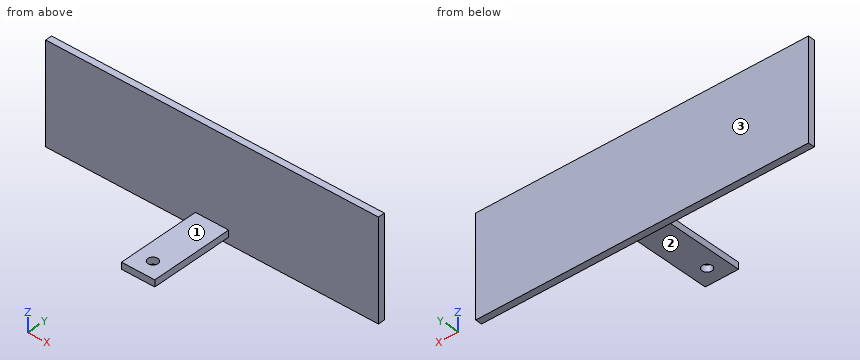
```python
from build123d import *

# Parameters (mm, degrees)
SKETCH1_W               = 2
SKETCH1_H               = 25
BOSS_EXTRUDE1_DEPTH     = 5
BOSS_EXTRUDE2_DEPTH     = 50
CUT_EXTRUDE1_DEPTH      = 64.348243859
CUT_EXTRUDE1_DEPTH_BACK = 64.348243859
SKETCH2_R               = 1.5


with BuildPart() as part:
    # Sketch1 → Boss-Extrude1 (new, symmetric)
    with BuildSketch(Plane(origin=(0, 0, 0), x_dir=(0, 0, -1), z_dir=(1, 0, 0))):
        with Locations((-1, 12.5)):
            Rectangle(SKETCH1_W, SKETCH1_H)
        Polygon((-2, 25), (-28, 25), (-28, 27), (2, 27), (2, 25), (0, 25), align=None)
    extrude(amount=BOSS_EXTRUDE1_DEPTH, both=True)

    # Sketch1_3 → Boss-Extrude2 (add, symmetric)
    with BuildSketch(Plane(origin=(0, 0, 0), x_dir=(0, 0, -1), z_dir=(1, 0, 0))):
        Polygon((-2, 25), (0, 25), (2, 25), (2, 27), (-28, 27), (-28, 25), align=None)
    extrude(amount=BOSS_EXTRUDE2_DEPTH, both=True)

    # Sketch2 → Cut-Extrude1 (cut, two sides: drawn at the far end of the back side and taken through both)
    with BuildSketch(Plane(origin=(0, 0, 0), x_dir=(-1, 0, 0), z_dir=(0, 0, -1)).offset(-CUT_EXTRUDE1_DEPTH_BACK)):
        with Locations((0, 5)):
            Circle(SKETCH2_R)
    extrude(amount=CUT_EXTRUDE1_DEPTH + CUT_EXTRUDE1_DEPTH_BACK, mode=Mode.SUBTRACT)


solid = part.part
```
CAD build for the part. Positions are in the model's coordinates, mm. Face numbers are marked on the shaded views. A direction names the side the tool comes from. Round coordinates to 2 decimals unless told otherwise and drop trailing zeros. Loops run counter-clockwise (first coordinate to the right, second up) from the corner with the lowest first, then second, coordinate; pieces in that order, holes last. Notation, with made-up numbers: M 55.5,-30 L 104.5,-30 A23 cw 104.5,5 Z; hole C -10,-34 d3. An arc over 180 degrees is marked long. Return JSON: item names as keys, results as strings. Group by question number.
(1) Saw through at A-A, the plane y = 5. List the corners of the cut face in (x, z).
(2) Drop flat-ended pins along their axis: P1, Ø3, axis at x = -1.5, y = 7.5, coming from the -Z side; P2, Ø9, axis at x = 14, z = 15.5, coming from the -Y side; P3, Ø4, axis at x = -0.5, y = 7, coming from the +Z side. Give the stop position or say it passes through.
(3) Saw through at C-C, the plane y = 9.5. List the corners of the cut face in (x, z).
(4) Saw through at B-B, the plane x = 0. List the corners of the cut face in (y, z).
(5) Wall check: probe 1 along X at (y, z) = (5, 1.25); probe 2 along Y at (x, z) = (0, 0.7); probe 3 along Y at (x, z) = (0, 14.5). Give the ranges that are in metal, low to high. Write a range as [from, to].
(6) Saw through at D-D, the plane z = 16. List the corners of the cut face in (x, y).
(7) Tool access for the marked faces 1, 2 and 3: list every direction of +Z, -Z, +X, -X, +Y, -Y with a clear straight run to the whole face (end or side of a thin tool).
Answer list:
{
 "1": {"outline": "M -5,0 L -1.5,0 L -1.5,2 L -5,2 Z; M 1.5,0 L 5,0 L 5,2 L 1.5,2 Z"},
 "2": {"P1": "z = 0", "P2": "y = 25", "P3": "z = 2"},
 "3": {"outline": "M -5,0 L 5,0 L 5,2 L -5,2 Z"},
 "4": {"outline": "M 0,0 L 3.5,0 L 3.5,2 L 0,2 Z; M 6.5,0 L 25,0 L 25,-2 L 27,-2 L 27,28 L 25,28 L 25,2 L 6.5,2 Z"},
 "5": {"probe 1": "[-5, -1.5], [1.5, 5]", "probe 2": "[0, 3.5], [6.5, 27]", "probe 3": "[25, 27]"},
 "6": {"outline": "M -50,25 L 50,25 L 50,27 L -50,27 Z"},
 "7": {"face 1": "+Z, +X, -X, -Y", "face 2": "-Z, +X, -X, -Y", "face 3": "+Z, -Z, +X, -X, +Y"}
}
